Print and shaded views of the part. All mm, measured from the part's lowest x, y and z. A direction names the side the tool comes from. Give positions to 0.01 mm unless a question says otherwise; leave off trailing zeros. Write each loop counter-clockwise with the first axis right and the second up, starting at its lowest first coordinate (ties: lowest second). Pieces come first, ordered by that corner, then holes. Notation, with made-up numbers: (80, 74.25) -> (107, 74.25) arc R31 cw to (107, 103.25) -> close; hole circle Ø8 at (22, 64). An arc over 180 degrees is marked (long way). Put each result on its own line as item: value.
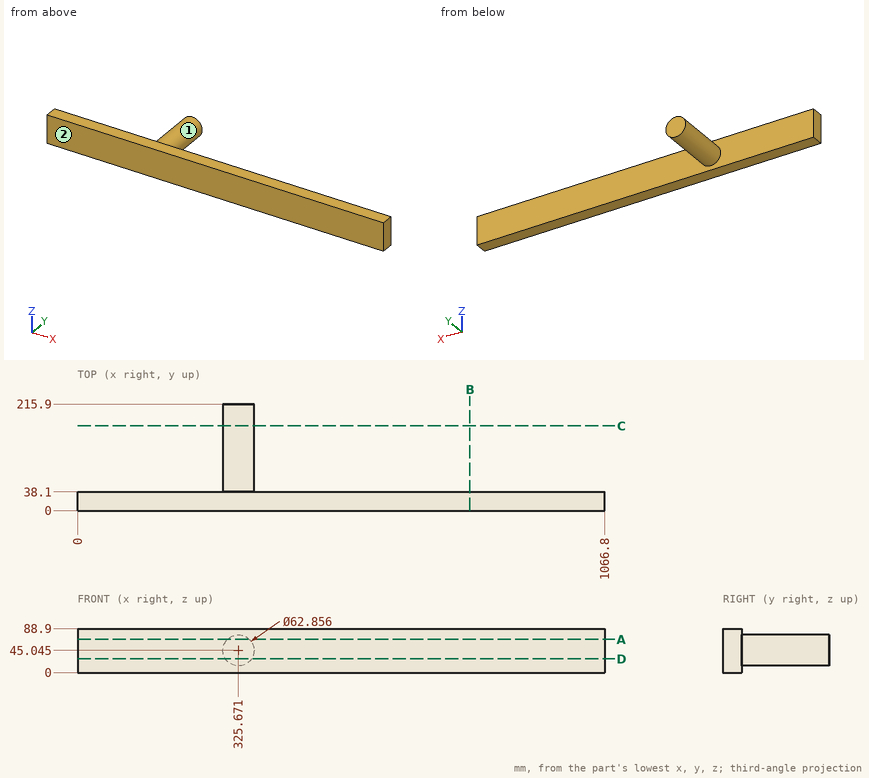
1) Slice it at B-B (x = 794). Write the cut outline in (y, z), plus the area to 3 significant figures.
Filled sheet:
outline: (0, 0) -> (38.1, 0) -> (38.1, 88.9) -> (0, 88.9) -> close
area: 3,390 mm2
2) Slice it at D-D (z = 28). Write the cut outline in (x, y) (1 decimal).
Filled sheet:
outline: (0, 0) -> (1066.8, 0) -> (1066.8, 38.1) -> (352.1, 38.1) -> (352.1, 215.9) -> (299.3, 215.9) -> (299.3, 38.1) -> (0, 38.1) -> close
3) Slice it at A-A (z = 67.5). Write the cut outline in (x, y).
Filled sheet:
outline: (0, 0) -> (1066.8, 0) -> (1066.8, 38.1) -> (347.66, 38.1) -> (347.66, 215.9) -> (303.68, 215.9) -> (303.68, 38.1) -> (0, 38.1) -> close
4) Tool access for the marked faces 1 and 2: list every direction of +Z, -Z, +X, -X, +Y, -Y with a clear straight run to the whole face (end or side of a thin tool).
Filled sheet:
face 1: +Y
face 2: +Z, -Z, +X, -X, -Y
5) Slice it at C-C (y = 171.5). Write the cut outline in (x, z) (1 decimal).
Filled sheet:
outline: circle Ø62.9 at (325.7, 45)
6) Pin check, flat tips, straight feed: pin 1 (6 mm diameter, centred on y = 148, z = 56, fed in from -X); pin 2 (8 mm diameter, centred on y = 117.5, z = 33.5, fed in from -X); pin 3 (3 mm diameter, centred on x = 347.5, y = 118.5, fed in from +Z). Stop position of each tip, or through.
Filled sheet:
pin 1: x = 295.27
pin 2: x = 295.16
pin 3: z = 69.01
7) Wall check: L1, parallel to Y at x = 524, z = 85.5; L2, parallel to Z at x = 324, y = 105; L3, parallel to X at y = 42, z = 60 (1 decimal). Give the ranges that are in metal, low to high.
Filled sheet:
L1: 0 to 38.1
L2: 13.66 to 76.43
L3: 298 to 353.3
